```python
from build123d import *

# Parameters (mm, degrees)
SKETCH1_R           = 50
BOSS_EXTRUDE1_DEPTH = 12.5


with BuildPart() as part:
    # Sketch1 → Boss-Extrude1 (new body)
    with BuildSketch(Plane.XY):
        with BuildLine():
            ThreePointArc((80.269796006, -12.90154445), (64.968632792, 0.106555165), (80.22704459, 13.164775589))
            Line((80.22704459, 13.164775589), (99.127347992, 13.182142467))
            ThreePointArc((99.127347992, 13.182142467), (70.645692195, 70.775604372), (13, 99.151399385))
            Line((13, 99.151399385), (12.998692028, 82.58389221))
            ThreePointArc((12.998692028, 82.58389221), (1.164991508, 68.412255439), (-13, 80.253909562))
            ThreePointArc((-13, 80.253909562), (-13.051446481, 81.411603502), (-13, 82.569297441))
            Line((-13, 82.569297441), (-13, 99.151399385))
            ThreePointArc((-13, 99.151399385), (-70.710695757, 70.71066048), (-99.151405871, 12.999950534))
            Line((-99.151405871, 12.999950534), (-80.251102468, 13.017317412))
            ThreePointArc((-80.251102468, 13.017317412), (-67.29756358, 0.062140866), (-80.252740126, -12.891398023))
            Line((-80.252740126, -12.891398023), (-99.165733386, -12.890202557))
            ThreePointArc((-99.165733386, -12.890202557), (-70.737321503, -70.684024692), (-12.964943151, -99.155989477))
            Line((-12.964943151, -99.155989477), (-12.984340134, -80.237755153))
            ThreePointArc((-12.984340134, -80.237755153), (0.009254017, -68.272284652), (12.985836125, -80.256202627))
            Line((12.985836125, -80.256202627), (12.984344225, -99.153450797))
            ThreePointArc((12.984344225, -99.153450797), (70.739768795, -70.681575469), (99.164103047, -12.902738735))
            Line((99.164103047, -12.902738735), (80.269796006, -12.90154445))
        make_face()
        Circle(SKETCH1_R, mode=Mode.SUBTRACT)
    extrude(amount=BOSS_EXTRUDE1_DEPTH)


solid = part.part
```
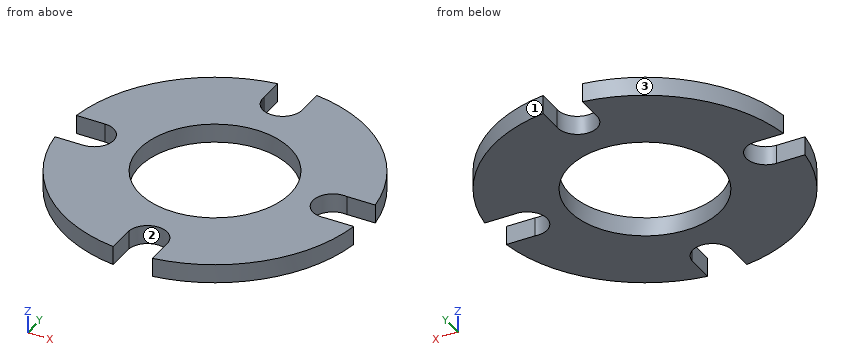
Read the model definition and answer for the solid it produces. Units are mm, in the model's axes. Face numbers are marked on the shaded views. Give positions to 0.01 mm unless a question says otherwise; leave off trailing zeros. Loops run counter-clockwise (first coordinate to the right, second up) from the corner with the lowest first, then second, coordinate; pieces in that order, holes last.
Item 1: Find the intervals of material crossed by line 1 along Y through (x, z) = (0, 8.5); line 2 along Y through (x, z) = (22.5, 1.5); line 3 along X through (y, z) = (81.5, 8.25), in increasing order.
Item 2: The part is cut by section D-D (x = -53). Write down the section's boundary in (y, z), and give its area (3 significant figures).
Item 3: The part is cut by section A-A (x = 0). Write down the section's boundary in (y, z).
Item 4: Each of these flat-tipped pins is pushed along its axis until it touches: pin 1 Ø6 at (x, z) = (7.5, 6) entering from -Y; pin 2 Ø1 at (x, z) = (7.5, 8.5) entering from -Y; pin 3 Ø6 at (x, z) = (86.5, 5.5) entering from +Y (3 decimals). Where does it stop, or does it pass through?
Item 5: The part is cut by section B-B (z = 5.5). Write down the section's boundary in (x, y).
Item 6: The part is cut by section C-C (y = 0). Write down the section's boundary in (x, z).
Item 7: The mould has two halves that part along X. Classify the marked faces 1, 2 and 3: released by +X, released by -X, zero draft, split by the parting line, or undercut.
Taken from the geometry:
1. line 1: y = -68.27 to -50, 50 to 68.36
1. line 2: y = -97.44 to -44.65, 44.65 to 97.44
1. line 3: x = -57.95 to -13.05, 13.05 to 57.95
2. outline: (-84.8, 0) - (84.8, 0) - (84.8, 12.5) - (-84.8, 12.5) - close
2. area: 2,120 mm2
3. outline: (-68.27, 0) - (-50, 0) - (-50, 12.5) - (-68.27, 12.5) - close; (50, 0) - (68.36, 0) - (68.36, 12.5) - (50, 12.5) - close
4. pin 1: stops at y = -73.59
4. pin 2: stops at y = -71.02
4. pin 3: stops at y = 55.025
5. outline: (-99.17, -12.89) arc R100 ccw to (-12.96, -99.16) - (-12.98, -80.24) arc R13.03 cw to (12.99, -80.26) - (12.98, -99.15) arc R100 ccw to (99.16, -12.9) - (80.27, -12.9) arc R13.2 cw (long way) to (80.23, 13.16) - (99.13, 13.18) arc R100 ccw to (13, 99.15) - (13, 82.58) arc R13.05 cw (long way) to (-13, 82.57) - (-13, 99.15) arc R100 ccw to (-99.15, 13) - (-80.25, 13.02) arc R12.95 cw to (-80.25, -12.89) - close; hole circle Ø100 at (0, 0)
6. outline: (-67.3, 0) - (-50, 0) - (-50, 12.5) - (-67.3, 12.5) - close; (50, 0) - (64.97, 0) - (64.97, 12.5) - (50, 12.5) - close
7. face 1: released by +X
7. face 2: undercut
7. face 3: released by -X
